Autodesk Inventor part; units mm, degrees
ref_plane "YZ Plane" through (0, 0, 0) normal (1, 0, 0) x (0, 1, 0)
ref_plane "XZ Plane" through (0, 0, 0) normal (0, 1, 0) x (-1, 0, 0)
ref_plane "XY Plane" through (0, 0, 0) normal (0, 0, 1) x (1, 0, 0)
sketch "Sketch1" plane through (0, 0, 0) normal (0, 0, 1) x (1, 0, 0)
  line L0 (-64.77, 64.77) -> (64.77, 64.77)
  line L1 (64.77, 64.77) -> (64.77, -64.77)
  line L2 (64.77, -64.77) -> (-64.77, -64.77)
  line L3 (-64.77, -64.77) -> (-64.77, 64.77)
  line L4 (-64.77, 64.77) -> (64.77, -64.77) construction
  line L5 (64.77, 64.77) -> (-64.77, -64.77) construction
  point P0 (0, 0)
  dimension "d0" = 129.54
extrude "Extrusion1" add sketch "Sketch1" along normal blind 50.8
shell "Shell1" thickness 3.175 outward yes removed faces 1 at (-21.59, -21.59, 50.8)
sketch "Sketch2" plane through (0, 0, 0) normal (0, 0, 1) x (1, 0, 0)
  line L0 (-67.945, 67.945) -> (-67.945, -67.945)
  circle A0 centre (-67.945, 67.945) radius 4.7752
  line L1 (67.945, -67.945) -> (67.945, 67.945)
  circle A1 centre (67.945, 67.945) radius 4.7752
  line L2 (-67.945, -67.945) -> (67.945, -67.945)
  circle A2 centre (67.945, -67.945) radius 4.7752
  circle A3 centre (-67.945, -67.945) radius 4.7752
  point P0 (0, 0)
  dimension "d4" = 9.5504
extrude "Extrusion2" add sketch "Sketch2" along normal blind 50.8 and the other way blind 3.175
sketch "Sketch3" plane through (0, 0, 50.8) normal (0, 0, 1) x (1, 0, 0)
  line L0 (-67.945, 63.1698) -> (-67.945, -63.1698)
  circle A0 centre (-67.945, -67.945) radius 1.7996
  line L1 (-63.1698, -67.945) -> (63.1698, -67.945)
  arc A1 (-67.945, -63.1698) -> (-63.1698, -67.945) centre (-67.945, -67.945) ccw
  arc A2 (-63.1698, 67.945) -> (-67.945, 63.1698) centre (-67.945, 67.945) ccw
  circle A3 centre (-67.945, 67.945) radius 1.7996
  arc A4 (67.945, 63.1698) -> (63.1698, 67.945) centre (67.945, 67.945) ccw
  circle A5 centre (67.945, 67.945) radius 1.7996
  arc A6 (63.1698, -67.945) -> (67.945, -63.1698) centre (67.945, -67.945) ccw
  circle A7 centre (67.945, -67.945) radius 1.7996
  point P0 (0, 0)
  point P1 (82.55, 82.55)
  dimension "d17" = 3.5992
extrude "Extrusion3" cut sketch "Sketch3" along normal mid plane 107.95
sketch "Sketch4" plane through (-63.1698, 67.945, -3.175) normal (0, 1, 0) x (1, 0, 0)
  line L0 (44.1198, -19.939) -> (82.2198, -19.939)
  line L1 (82.2198, -19.939) -> (82.2198, -42.545)
  line L2 (82.2198, -42.545) -> (44.1198, -42.545)
  line L3 (44.1198, -42.545) -> (44.1198, -19.939)
  line L4 (44.1198, -19.939) -> (82.2198, -42.545) construction
  line L5 (82.2198, -19.939) -> (44.1198, -42.545) construction
  line L6 (126.3396, -53.975) -> (0, -53.975)
  point P0 (63.1698, -3.175)
  point P1 (63.1698, -31.242)
  point P2 (63.1698, -31.242)
  point P3 (160.9128, -53.975)
  point P4 (-0.588, -53.975)
  dimension "d12" = 38.1
  dimension "d13" = 22.606
  dimension "d14" = 11.43
extrude "Extrusion4" cut sketch "Sketch4" against normal up to next
properties part number "PS-01" material "Aluminum 6061(1)"
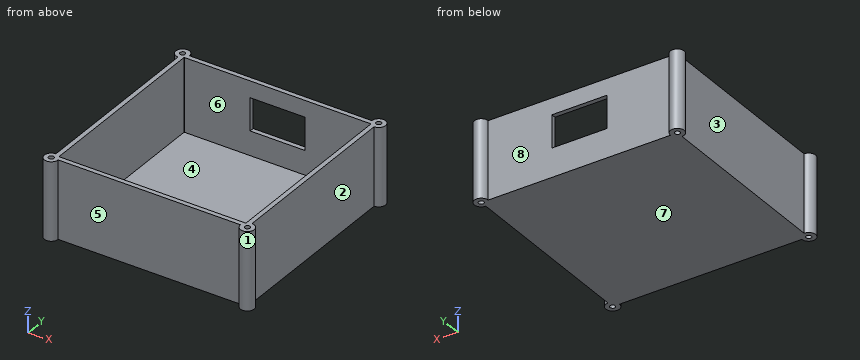
Build history of the part. All positions in model axes, mm. Face numbers are marked on the shaded views. A direction names the side the tool comes from. Round coordinates to 2 decimals unless told otherwise and drop trailing zeros. Loops run counter-clockwise (first coordinate to the right, second up) from the corner with the lowest first, then second, coordinate; pieces in that order, holes last. Notation, with made-up numbers: (13.25, 68) -> (45.25, 68) arc R24 cw to (45.25, 81) -> close; hole circle Ø11 at (83.25, 49). An arc over 180 degrees is marked (long way). Use CSV: the item, a comma, the result in double quotes. Start each with the question number.
Q1. Saw through at B-B on z = 46. Give the cut face in (x, y) (3 decimals), and give its area (3 significant figures).
Q2. Drill centre lines: L1, parallel to X at y = 0.5, z = 39.5 (3 decimals); L2, parallel to Y at x = 10, z = 26 (3 decimals). Where is each one in solid material? Low to high.
Q3. Flat gauge pins, fed straight in: pin 1 Ø1 at (x, z) = (-33.5, 3) entering from +Y (3 decimals); pin 2 Ø4 at (y, z) = (49, 14) entering from -X (3 decimals); pin 3 Ø10 at (x, z) = (-41.5, 23.5) entering from -Y (3 decimals); pin 4 Ø4 at (x, y) = (-67.945, -67.945) entering from -Z (3 decimals). Where does each tip first touch, or does it go through?
Q4. Saw through at D-D on y = -0.5. Give the cut face in (x, z) (3 decimals), and give its area (3 significant figures).
Q5. Mould opens along Y. For the marked faces 5, 6, 7 and 8 say: +Y half, -Y half, draft (parallel to the pull), parting line (faces both ways), or undercut.
Q6. Saw through at A-A on x = -13.5. Give the cut face in (y, z) (3 decimals).
Q7. Which spindle directions (+Z, -Z, +X, -X, +Y, -Y) get a long thin tool onto all of the face, cutting with end or side? Do the marked faces 1, 2, 3 and 4. Say none if no direction does.
Q8. Saw through at C-C on z = 35. Give the cut face in (x, y) (3 decimals).
Solutions:
1,outline,"(-67.945, -63.17) arc R4.775 ccw (long way) to (-63.17, -67.945) -> (63.17, -67.945) arc R4.775 ccw (long way) to (67.945, -63.17) -> (67.945, 63.17) arc R4.775 ccw (long way) to (63.17, 67.945) -> (-63.17, 67.945) arc R4.775 ccw (long way) to (-67.945, 63.17) -> close; hole circle Ø3.599 at (-67.945, -67.945); hole circle Ø3.599 at (-67.945, 67.945); hole (-64.77, -64.378) arc R4.775 cw to (-64.378, -64.77) -> (64.378, -64.77) arc R4.775 cw to (64.77, -64.378) -> (64.77, 64.378) arc R4.775 cw to (64.378, 64.77) -> (-64.378, 64.77) arc R4.775 cw to (-64.77, 64.378) -> close; hole circle Ø3.599 at (67.945, -67.945); hole circle Ø3.599 at (67.945, 67.945)"
1,area,"1,860 mm^2"
2,L1,"x = -67.945 to -64.77, 64.77 to 67.945"
2,L2,"y = -67.945 to -64.77"
3,pin 1,"stops at y = 67.945"
3,pin 2,"stops at x = -67.945"
3,pin 3,"stops at y = -67.945"
3,pin 4,"stops at z = -3.175"
4,outline,"(-67.945, -3.175) -> (67.945, -3.175) -> (67.945, 50.8) -> (64.77, 50.8) -> (64.77, 0) -> (-64.77, 0) -> (-64.77, 50.8) -> (-67.945, 50.8) -> close"
4,area,"754 mm^2"
5,face 5,"-Y half"
5,face 6,"undercut"
5,face 7,"draft"
5,face 8,"+Y half"
6,outline,"(-67.945, -3.175) -> (67.945, -3.175) -> (67.945, 16.764) -> (64.77, 16.764) -> (64.77, 0) -> (-64.77, 0) -> (-64.77, 50.8) -> (-67.945, 50.8) -> close; (64.77, 39.37) -> (67.945, 39.37) -> (67.945, 50.8) -> (64.77, 50.8) -> close"
7,face 1,"+Z, -Z"
7,face 2,"+Z, -Z, +X"
7,face 3,"+Z, -Z, -X"
7,face 4,"+Z"
8,outline,"(-67.945, -63.17) arc R4.775 ccw (long way) to (-63.17, -67.945) -> (63.17, -67.945) arc R4.775 ccw (long way) to (67.945, -63.17) -> (67.945, 63.17) arc R4.775 ccw (long way) to (63.17, 67.945) -> (19.05, 67.945) -> (19.05, 64.77) -> (64.378, 64.77) arc R4.775 ccw to (64.77, 64.378) -> (64.77, -64.378) arc R4.775 ccw to (64.378, -64.77) -> (-64.378, -64.77) arc R4.775 ccw to (-64.77, -64.378) -> (-64.77, 64.378) arc R4.775 ccw to (-64.378, 64.77) -> (-19.05, 64.77) -> (-19.05, 67.945) -> (-63.17, 67.945) arc R4.775 ccw (long way) to (-67.945, 63.17) -> close; hole circle Ø3.599 at (-67.945, -67.945); hole circle Ø3.599 at (-67.945, 67.945); hole circle Ø3.599 at (67.945, -67.945); hole circle Ø3.599 at (67.945, 67.945)"
